from build123d import *

# Parameters (mm, degrees)
SKETCH1_R           = 4
BOSS_EXTRUDE1_DEPTH = 5.2
SKETCH2_OUTSIDE_W   = 38.002
SKETCH2_OUTSIDE_H   = 36.038
SKETCH2_OUTSIDE_R   = 6.35
CUT_EXTRUDE1_DEPTH  = 5
CUT_EXTRUDE1_TAPER  = 60
SKETCH3_OUTSIDE_W   = 38.002
SKETCH3_OUTSIDE_H   = 36.038
SKETCH3_OUTSIDE_R   = 6.35
CUT_EXTRUDE2_DEPTH  = 5
CUT_EXTRUDE2_TAPER  = 60


with BuildPart() as part:
    # Sketch1 → Boss-Extrude1 (new body)
    with BuildSketch(Plane.XY):
        Polygon((7.332348419, 0), (3.666174209, 6.35), (-3.666174209, 6.35), (-7.332348419, 0), (-3.666174209, -6.35), (3.666174209, -6.35), align=None)
        Circle(SKETCH1_R, mode=Mode.SUBTRACT)
    extrude(amount=BOSS_EXTRUDE1_DEPTH)

    # Sketch2 outside → Cut-Extrude1 (cut)
    with BuildSketch(Plane.XY.offset(5.2)):
        Rectangle(SKETCH2_OUTSIDE_W, SKETCH2_OUTSIDE_H)
        Circle(SKETCH2_OUTSIDE_R, mode=Mode.SUBTRACT)
    extrude(amount=-CUT_EXTRUDE1_DEPTH, taper=CUT_EXTRUDE1_TAPER, mode=Mode.SUBTRACT)

    # Sketch3 outside → Cut-Extrude2 (cut)
    with BuildSketch(Plane(origin=(0, 0, 0), x_dir=(-1, 0, 0), z_dir=(0, 0, -1))):
        Rectangle(SKETCH3_OUTSIDE_W, SKETCH3_OUTSIDE_H)
        Circle(SKETCH3_OUTSIDE_R, mode=Mode.SUBTRACT)
    extrude(amount=-CUT_EXTRUDE2_DEPTH, taper=CUT_EXTRUDE2_TAPER, mode=Mode.SUBTRACT)


solid = part.part
Model file for the job. Use its own axes, mm. Round coordinates to 2 decimals unless told otherwise and drop trailing zeros. Loops run counter-clockwise (first coordinate to the right, second up) from the corner with the lowest first, then second, coordinate; pieces in that order, holes last.
1. Wall check: probe 1 along Y at (x, z) = (0, 1.4); probe 2 along Y at (x, z) = (1.75, 1.7); probe 3 along X at (y, z) = (0.75, 0.9). Give the ranges that are in metal, low to high.
Check values:
probe 1: y = -6.35 to -4, 4 to 6.35
probe 2: y = -6.35 to -3.6, 3.6 to 6.35
probe 3: x = -6.9 to -3.93, 3.93 to 6.9
2. Mould opens along Y. For faces 1 (the flat face through (0, 6.35, 3)), 2 (the cylindrical face through (-0.867, -3.905, 2.564)), 3 (the conical face through (-3.28, -5.714, 5.062)) say: +Y half, -Y half, draft (parallel to the pull), parting line (faces both ways), or undercut.
Check values:
face 1: +Y half
face 2: undercut
face 3: -Y half
3. Band-saw the part on A-A, the plane z = 3.7. List the corners of the cut face in (x, y).
Check values:
outline: (-7.33, 0) - (-3.67, -6.35) - (3.67, -6.35) - (7.33, 0) - (3.67, 6.35) - (-3.67, 6.35) - close; hole circle Ø8 at (0, 0)
4. Drop a flat-ended pin along its axis: P1, Ø1, axis at x = 5.5, z = 3, coming from the +Y side. Give the stop position or say it passes through.
Check values:
P1: stops at y = 4.04
